Build history of the part. All positions in model axes, mm. Face numbers are marked on the shaded views. A direction names the side the tool comes from. Give positions to 0.01 mm unless a question says otherwise; leave off trailing zeros. Loops run counter-clockwise (first coordinate to the right, second up) from the corner with the lowest first, then second, coordinate; pieces in that order, holes last. Notation, with made-up numbers: (10.25, 46.25) -> (52.25, 46.25) arc R5 ccw to (52.25, 55.25) -> close; hole circle Ø11 at (66, 18.25). An arc over 180 degrees is marked (long way). Answer as a JSON object with one key per item and string values. Group by question number.
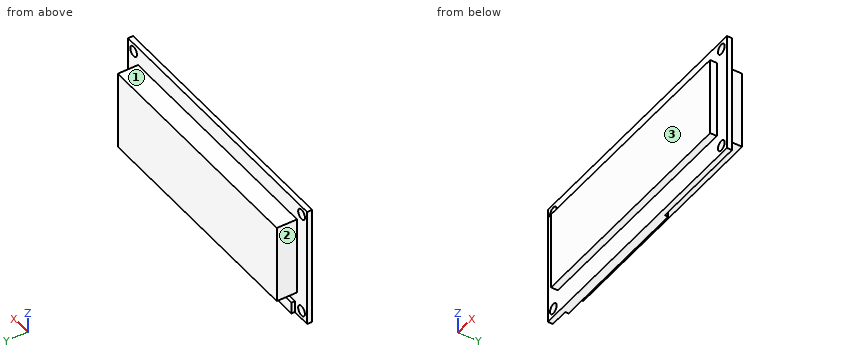
from build123d import *

# Parameters (mm, degrees)
SKETCH_1_W            = 80
SKETCH_1_H            = 36
SKETCH_1_R            = 1.5
EXTRUDE_1_DEPTH       = 1.5
EXTRUDE_START         = 7
EXTRUDE_2_OUTLINE_W   = 71
EXTRUDE_2_OUTLINE_H   = 6
EXTRUDE_2_OUTLINE_H_2 = 2
EXTRUDE_2_DEPTH       = 23.5
EXTRUDE_2_2_OUTLINE_W = 44.5
EXTRUDE_2_2_OUTLINE_H = 1
EXTRUDE_2_2_DEPTH     = 3.5


# Read off the part's stored shape, not the designer's step: Бобышка-Вытянуть2
with BuildPart() as part:
    # Эскиз1 (on Top Plane) → Бобышка-Вытянуть1 (new body)
    with BuildSketch(Plane(origin=(0, 0, 0), x_dir=(1, 0, 0), z_dir=(0, 1, 0))):
        with Locations((40, -18)):
            Rectangle(SKETCH_1_W, SKETCH_1_H)
        with Locations(Location((2.5, -2.5, 0), (0, 0, 270))):
            Circle(SKETCH_1_R, mode=Mode.SUBTRACT)
        with Locations(Location((77.5, -2.5, 0), (0, 0, 90))):
            Circle(SKETCH_1_R, mode=Mode.SUBTRACT)
        with Locations(Location((77.5, -33.5, 0), (0, 0, 270))):
            Circle(SKETCH_1_R, mode=Mode.SUBTRACT)
        with Locations(Location((2.5, -33.5, 0), (0, 0, 90))):
            Circle(SKETCH_1_R, mode=Mode.SUBTRACT)
    extrude(amount=EXTRUDE_1_DEPTH)

    # Бобышка-Вытянуть2 outline → Бобышка-Вытянуть2 (add)
    with BuildSketch(Plane.XY.offset(EXTRUDE_START)):
        with Locations((40, 4.5)):
            Rectangle(EXTRUDE_2_OUTLINE_W, EXTRUDE_2_OUTLINE_H)
        with Locations((40, -1)):
            Rectangle(EXTRUDE_2_OUTLINE_W, EXTRUDE_2_OUTLINE_H_2)
    extrude(amount=EXTRUDE_2_DEPTH)

    # Extrude 2 2 outline → Extrude 2 2 (add)
    with BuildSketch(Plane.XY):
        with Locations((27.75, 2)):
            Rectangle(EXTRUDE_2_2_OUTLINE_W, EXTRUDE_2_2_OUTLINE_H)
    extrude(amount=EXTRUDE_2_2_DEPTH)


solid = part.part
(1) Saw through at C-C on x = 9. List the corners of the cut face in (y, z).
(2) Saw through at A-A on z = 2.5. List the corners of the cut face in (x, y).
(3) Saw through at D-D on z = 14.5. List the corners of the cut face in (x, y).
(4) Probe line 1 along X through (y, z) = (0.4, 2.5); line 2 along Z through (x, y) = (77.5, 0.7); line 3 along Y through (x, z) = (39, 6). List the from-to ranges inside material, lowest first. Write a range as [from, to].
(5) Saw through at B-B on x = 77.5. List the corners of the cut face in (y, z), plus the area to 3 significant figures.
(6) 3-axis set-ups, long thin cutter, end or side, ignore diameter. For the marked faces 1, 2 and 3: which of +Z, -Z, +X, -X, +Y, -Y reach the whole face in a straight line?
(7) Pin check, flat tips, straight feed: pin 1 (2 mm diameter, centred on x = 31.5, y = 4, fed in from +Z); pin 2 (0.8 mm diameter, centred on y = 2, z = 1, fed in from -X); pin 3 (1.6 mm diameter, centred on y = -1, z = 23.5, fed in from +X). Stop position of each tip, or through.
Calculated:
{
 "1": {"outline": "(-2, 7) -> (0, 7) -> (0, 0) -> (2.5, 0) -> (2.5, 3.5) -> (1.5, 3.5) -> (1.5, 7) -> (7.5, 7) -> (7.5, 30.5) -> (1.5, 30.5) -> (1.5, 36) -> (0, 36) -> (0, 30.5) -> (-2, 30.5) -> close"},
 "2": {"outline": "(0, 0) -> (1, 0) -> (1, 1.5) -> (0, 1.5) -> close; (4, 0) -> (76, 0) -> (76, 1.5) -> (50, 1.5) -> (50, 2.5) -> (5.5, 2.5) -> (5.5, 1.5) -> (4, 1.5) -> close; (79, 0) -> (80, 0) -> (80, 1.5) -> (79, 1.5) -> close"},
 "3": {"outline": "(0, 0) -> (4.5, 0) -> (4.5, -2) -> (75.5, -2) -> (75.5, 0) -> (80, 0) -> (80, 1.5) -> (75.5, 1.5) -> (75.5, 7.5) -> (4.5, 7.5) -> (4.5, 1.5) -> (0, 1.5) -> close"},
 "4": {"line 1": "x = [0, 1], [4, 76], [79, 80]", "line 2": "z = [0, 1], [4, 32], [35, 36]", "line 3": "y = [0, 1.5]"},
 "5": {"outline": "(0, 0) -> (1.5, 0) -> (1.5, 1) -> (0, 1) -> close; (0, 4) -> (1.5, 4) -> (1.5, 32) -> (0, 32) -> close; (0, 35) -> (1.5, 35) -> (1.5, 36) -> (0, 36) -> close", "area": "45.0 mm^2"},
 "6": {"face 1": "+Z, +X, -X, +Y", "face 2": "+Z, -Z, -X, +Y", "face 3": "+Z, -Z, +X, -X, -Y"},
 "7": {"pin 1": "stops at z = 30.5", "pin 2": "stops at x = 5.5", "pin 3": "stops at x = 75.5"}
}
